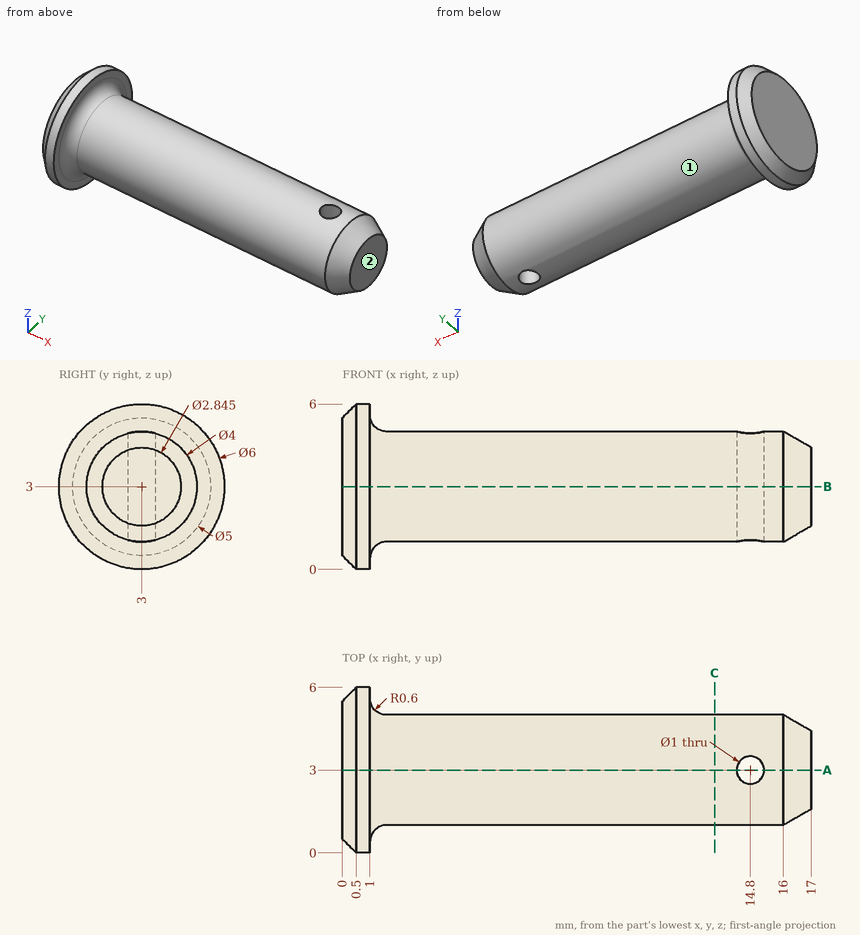
Source: three-view drawing plus pictorial views. Frame: mm from the lowest corner of the part. A direction names the side the tool comes from. Round coordinates to 2 decimals unless told otherwise and drop trailing zeros. Loops run counter-clockwise (first coordinate to the right, second up) from the corner with the lowest first, then second, coordinate; pieces in that order, holes last. Notation, with made-up numbers: (-31.5, 82.5) - (-18.5, 82.5) arc R34 ccw to (-18.5, 118.5) - close; hole circle Ø10 at (56, 82.25). An arc over 180 degrees is marked (long way). Write item = value, one per line. Start each with the question number.
Item 1: Section query A-A on y = 3. Output: boundary loops of the cut face in (x, z).
Item 2: Section query B-B on z = 3. Output: boundary loops of the cut face in (x, y).
Item 3: Reachability of the marked faces 1 and 2 from +Z, -Z, +X, -X, +Y, -Y: full face, straight path, thin tool, end or side. Return the list, or none.
Item 4: Material intervals for line 1 (X direction, y = 3, z = 2); line 2 (Y direction, x = 5.25, z = 3.05); line 3 (Y direction, x = 14.8, z = 2.6), sorted ascending.
Item 5: First-contact query: pin 1 Ø2 at (x, y) = (11, 5) entering from +Z; pin 2 Ø1.5 at (x, z) = (5.5, 3.5) entering from +Y. Flat tips, straight axial feed; report the tip coordinate or a pass-through.
Item 6: Section query C-C on x = 13.5. Output: boundary loops of the cut face in (y, z).
Results list:
q1.outline = (0, 0.5) - (0.5, 0) - (1, 0) - (1, 0.4) arc R0.6 cw to (1.6, 1) - (14.3, 1) - (14.3, 5) - (1.6, 5) arc R0.6 cw to (1, 5.6) - (1, 6) - (0.5, 6) - (0, 5.5) - close; (15.3, 1) - (16, 1) - (17, 1.58) - (17, 4.42) - (16, 5) - (15.3, 5) - close
q2.outline = (0, 0.5) - (0.5, 0) - (1, 0) - (1, 0.4) arc R0.6 cw to (1.6, 1) - (16, 1) - (17, 1.58) - (17, 4.42) - (16, 5) - (1.6, 5) arc R0.6 cw to (1, 5.6) - (1, 6) - (0.5, 6) - (0, 5.5) - close; hole circle Ø1 at (14.8, 3)
q3.face_1 = +X
q3.face_2 = +Z, -Z, +X, +Y, -Y
q4.line_1 = 0 to 14.3, 15.3 to 17
q4.line_2 = 1 to 5
q4.line_3 = 1.04 to 2.5, 3.5 to 4.96
q5.pin_1 = 4.73
q5.pin_2 = 5
q6.outline = circle Ø4 at (3, 3)
